For this review, use the dimensioned drawing (mm, ordinates from the lowest corner) and the shaded views. A direction names the side the tool comes from. Coordinates: 2 decimals unless noted, no trailing zeros. Order: outer loops, then holes, each group sorted by start corner. A loop starts at its lowest first (then second) coordinate and runs counter-clockwise, first axis right, second up. Notation, with made-up numbers: (4, 48.25) -> (11, 48.25) arc R11 cw to (11, 58.25) -> close; hole circle Ø8 at (87, -27). An arc over 180 degrees is marked (long way). Return JSON: item names as keys, results as strings. Group by question number.
Item 1: Insertion check: pin 1 (1.6 mm diameter, centred on y = 5, z = 7, fed in from +X); pin 2 (2 mm diameter, centred on x = 70, z = 3.5, fed in from -Y); pin 3 (4.5 mm diameter, centred on x = 30.5, y = 9.5, fed in from -Z); pin 4 (1 mm diameter, centred on y = 10, z = 6.5, fed in from +X). Each pin has a flat end and moves straight along its axis. Give the tip position at first contact, or say it passes through.
Item 2: Take a section at C-C (z = 4.75). Write out the cut boundary in (x, y).
Item 3: Take a section at A-A (y = 6). Write out the cut boundary in (x, z).
Item 4: Take a section at D-D (y = 2.8). Write out the cut boundary in (x, z).
Item 5: For line 1 along X through (y, z) = (3, 6.75); line 2 along Z through (x, y) = (4, 10); line 3 along Z through (x, y) = (32.5, 3), list the stretches that pass through material, from the lowest coordinate up.
Item 6: Take a section at B-B (x = 79). Write out the cut boundary in (y, z), then the cut area to 3 significant figures.
Item 7: Machinability: for the marked faces 1, 2 and 3, which of the approach directions +Z, -Z, +X, -X, +Y, -Y give a long, thin tool a straight path to every point of the face, cutting with its end or side? Answer none if there is none.
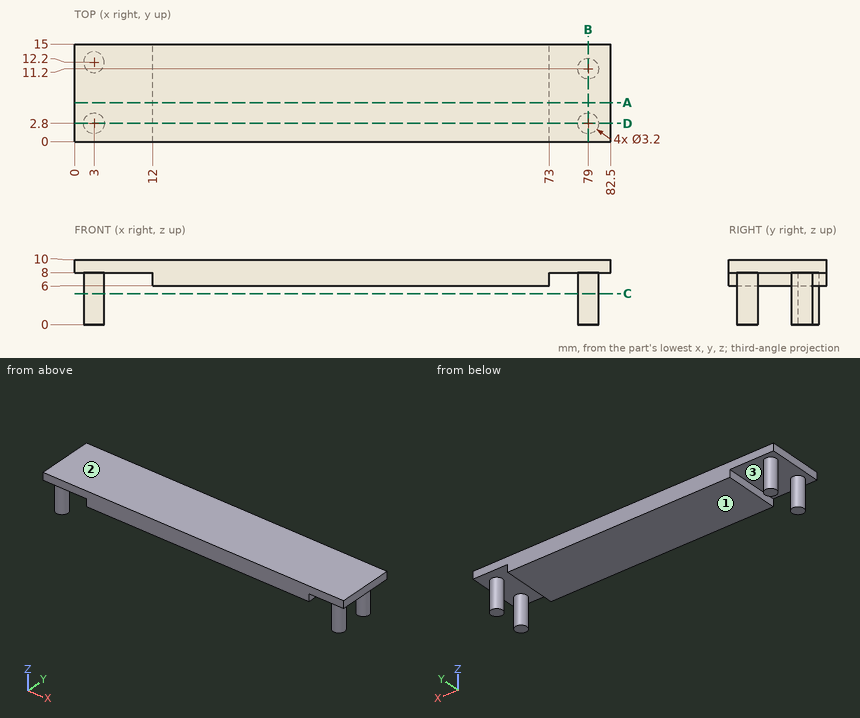
Findings below:
{
 "1": {"pin 1": "stops at x = 79.77", "pin 2": "passes through", "pin 3": "stops at z = 6", "pin 4": "stops at x = 80.44"},
 "2": {"outline": "circle Ø3.2 at (3, 2.8); circle Ø3.2 at (3, 12.2); circle Ø3.2 at (79, 2.8); circle Ø3.2 at (79, 11.2)"},
 "3": {"outline": "(0, 8) -> (12, 8) -> (12, 6) -> (73, 6) -> (73, 8) -> (82.5, 8) -> (82.5, 10) -> (0, 10) -> close"},
 "4": {"outline": "(0, 8) -> (1.4, 8) -> (1.4, 0) -> (4.6, 0) -> (4.6, 8) -> (12, 8) -> (12, 6) -> (73, 6) -> (73, 8) -> (77.4, 8) -> (77.4, 0) -> (80.6, 0) -> (80.6, 8) -> (82.5, 8) -> (82.5, 10) -> (0, 10) -> close"},
 "5": {"line 1": "x = 1.41 to 4.59, 12 to 73, 77.41 to 80.59", "line 2": "z = 8 to 10", "line 3": "z = 6 to 10"},
 "6": {"outline": "(0, 8) -> (1.2, 8) -> (1.2, 0) -> (4.4, 0) -> (4.4, 8) -> (9.6, 8) -> (9.6, 0) -> (12.8, 0) -> (12.8, 8) -> (15, 8) -> (15, 10) -> (0, 10) -> close", "area": "81.2 mm2"},
 "7": {"face 1": "-Z, +Y, -Y", "face 2": "+Z, +X, -X, +Y, -Y", "face 3": "-Z"}
}
